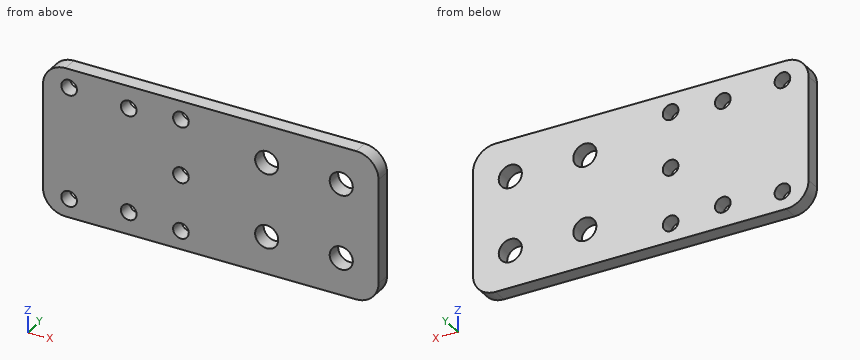
from build123d import *

# Parameters (mm, degrees)
SKETCH_1_W      = 45
SKETCH_1_H      = 20
SKETCH_1_R      = 1.55
SKETCH_1_R_2    = 1.05
EXTRUDE_1_DEPTH = 2
FILLET_1_R      = 3


with BuildPart() as part:
    # 草图1 → 凸台-拉伸1 (new body)
    with BuildSketch(Plane(origin=(0, 0, 0), x_dir=(1, 0, 0), z_dir=(0, 1, 0))):
        with Locations((22.5, 10)):
            Rectangle(SKETCH_1_W, SKETCH_1_H)
        with Locations(Location((30, 15, 0), (0, 0, 270))):
            Circle(SKETCH_1_R, mode=Mode.SUBTRACT)
        with Locations(Location((40, 15, 0), (0, 0, 270))):
            Circle(SKETCH_1_R, mode=Mode.SUBTRACT)
        with Locations(Location((40, 5, 0), (0, 0, 270))):
            Circle(SKETCH_1_R, mode=Mode.SUBTRACT)
        with Locations(Location((30, 5, 0), (0, 0, 270))):
            Circle(SKETCH_1_R, mode=Mode.SUBTRACT)
        with Locations(Location((11.5, 17, 0), (0, 0, 270))):
            Circle(SKETCH_1_R_2, mode=Mode.SUBTRACT)
        with Locations(Location((18.5, 10, 0), (0, 0, 270))):
            Circle(SKETCH_1_R_2, mode=Mode.SUBTRACT)
        with Locations(Location((11.5, 3, 0), (0, 0, 270))):
            Circle(SKETCH_1_R_2, mode=Mode.SUBTRACT)
        with Locations(Location((3.5, 17.5, 0), (0, 0, 270))):
            Circle(SKETCH_1_R_2, mode=Mode.SUBTRACT)
        with Locations(Location((18.5, 17.5, 0), (0, 0, 270))):
            Circle(SKETCH_1_R_2, mode=Mode.SUBTRACT)
        with Locations(Location((18.5, 2.5, 0), (0, 0, 270))):
            Circle(SKETCH_1_R_2, mode=Mode.SUBTRACT)
        with Locations(Location((3.5, 2.5, 0), (0, 0, 270))):
            Circle(SKETCH_1_R_2, mode=Mode.SUBTRACT)
    extrude(amount=EXTRUDE_1_DEPTH)

    # 圆角1
    fillet_1_edges = [part.edges().sort_by_distance(p)[0] for p in [
        (0, 1, -20),
        (45, 1, -20),
        (45, 1, 0),
        (0, 1, 0),
    ]]
    fillet(fillet_1_edges, radius=FILLET_1_R)


solid = part.part
Build history of the part. All positions in model axes, mm. Round coordinates to 2 decimals unless told otherwise and drop trailing zeros. Write each loop counter-clockwise with the first axis right and the second up, starting at its lowest first coordinate (ties: lowest second). Pieces come first, ordered by that corner, then holes. Notation, with made-up numbers: M -6,-31.5 L 38,-31.5 A23 cw 38,2.5 Z; hole C 45,39.25 d10. An arc over 180 degrees is marked long. Answer as a JSON object with one key per item and string values. Group by question number.
(1) Cut at B-B (x = 11.5). Give the cut face in (y, z).
(2) Cut at C-C (y = 1.2). Give the number of separate pieces and of enclosed holes in the cut face, and give its area (3 significant figures).
(3) Cut at A-A (z = -10). Give the cut face in (x, y).
(4) Drill centre lines: L1, parallel to X at y = 0.7, z = -15; L2, parallel to Z at x = 29, y = 1.45; L3, parallel to Z at x = 30.5, y = 0.75. Where is each one in solid material? Low to high.
(5) Cut at D-D (z = -6). Give the cut face in (x, y).
Responses:
{
 "1": {"outline": "M 0,-20 L 2,-20 L 2,-18.05 L 0,-18.05 Z; M 0,-15.95 L 2,-15.95 L 2,-4.05 L 0,-4.05 Z; M 0,-1.95 L 2,-1.95 L 2,0 L 0,0 Z"},
 "2": {"separate pieces": "1", "enclosed holes": "11", "area": "838 mm2"},
 "3": {"outline": "M 0,0 L 17.45,0 L 17.45,2 L 0,2 Z; M 19.55,0 L 45,0 L 45,2 L 19.55,2 Z"},
 "4": {"L1": "x = 0 to 28.45, 31.55 to 38.45, 41.55 to 45", "L2": "z = -20 to -16.18, -13.82 to -6.18, -3.82 to 0", "L3": "z = -20 to -16.47, -13.53 to -6.47, -3.53 to 0"},
 "5": {"outline": "M 0,0 L 28.82,0 L 28.82,2 L 0,2 Z; M 31.18,0 L 38.82,0 L 38.82,2 L 31.18,2 Z; M 41.18,0 L 45,0 L 45,2 L 41.18,2 Z"}
}
